Autodesk Inventor part; units mm, degrees
ref_plane "YZ Plane" through (0, 0, 0) normal (1, 0, 0) x (0, 1, 0)
ref_plane "XZ Plane" through (0, 0, 0) normal (0, 1, 0) x (-1, 0, 0)
ref_plane "XY Plane" through (0, 0, 0) normal (0, 0, 1) x (1, 0, 0)
sketch "Sketch1" plane through (0, 0, 0) normal (0, 0, 1) x (1, 0, 0)
  line L0 (-8.9, 0) -> (9.3, 0)
  line L1 (9.3, 0) -> (9.3, -14.13)
  line L2 (-8.9, -14.13) -> (-8.9, 0)
  line L3 (-7.7, -1.2) -> (8.1, -1.2)
  line L4 (8.1, -1.2) -> (8.1, -15.33)
  line L5 (-7.7, -15.33) -> (-7.7, -1.2)
  line L6 (-8.9, -14.13) -> (-17.7, -14.13)
  line L7 (-17.7, -14.13) -> (-17.7, -15.33)
  line L8 (-17.7, -15.33) -> (-7.7, -15.33)
  line L9 (9.3, -14.13) -> (18.1, -14.13)
  line L10 (18.1, -14.13) -> (18.1, -15.33)
  line L11 (18.1, -15.33) -> (8.1, -15.33)
  point P0 (0, 0)
  dimension "d0" = 1.2
  dimension "d1" = 1.2
  dimension "d2" = 1.2
  dimension "d3" = 15.8
  dimension "d4" = 14.13
  dimension "d5" = 10
  dimension "d6" = 10
  dimension "d7" = 1.2
  dimension "d8" = 1.2
extrude "Extrusion1" add sketch "Sketch1" along normal blind 10
sketch "Sketch2" plane through (-17.7, -14.13, 0) normal (0, 1, 0) x (1, 0, 0)
  line L0 (8.8, 0) -> (0, 0)
  line L1 (0, 0) -> (0, -10)
  line L2 (8.8, -10) -> (0, -10)
  line L3 (8.8, 0) -> (8.8, -10)
  point P0 (17.7, 0)
fillet "Fillet1" radius 1 2 edges at (18.1, -14.13, 5) (-17.7, -14.13, 5)
fillet "Fillet2" radius 1.5 4 edges at (-8.9, 0, 5) (9.3, 0, 5) (9.3, -14.13, 5) (-8.9, -14.13, 5)
sketch "Sketch3" plane through (-16.7, -14.13, 10) normal (0, 1, 0) x (1, 0, 0)
  circle A0 centre (3.15, 5) radius 0.5
  line L0 (33.8, 0) -> (27.5, 0)
  line L1 (27.5, 0) -> (27.5, 10)
  line L2 (33.8, 10) -> (27.5, 10)
  line L3 (33.8, 10) -> (33.8, 0)
  line L4 (27.5, 0) -> (27.5, 10)
  line L5 (33.8, 0) -> (27.5, 0)
  line L6 (33.8, 10) -> (33.8, 0)
  line L7 (33.8, 10) -> (27.5, 10)
  line L8 (34.8, 0) -> (33.8, 0)
  line L9 (33.8, 10) -> (34.8, 10)
  line L10 (34.8, 0) -> (34.8, 10)
  line L11 (33.8, 0) -> (34.8, 0)
  line L12 (34.8, 0) -> (34.8, 10)
  line L13 (34.8, 10) -> (33.8, 10)
  line L14 (33.8, 10) -> (33.8, 0)
  line L15 (34.8, 10) -> (34.8, 0)
  line L16 (34.8, 0) -> (34.8, 10)
  line L17 (34.8, 10) -> (34.8, 0)
  circle A1 centre (30.65, 5) radius 0.5
  point P0 (16.7, 10)
  dimension "d16" = 1
  dimension "d17" = 1
extrude "Extrusion2" cut sketch "Sketch3" against normal through all contours A0 | A1
properties part number "Batterijbevestiging"
Input: part model. Units: mm. Frame: model coordinates. A direction names the side the tool comes from. Give positions to 0.01 mm unless a question says otherwise; leave off trailing zeros. Loops run counter-clockwise (first coordinate to the right, second up) from the corner with the lowest first, then second, coordinate; pieces in that order, holes last.
1) Line query: L1, parallel to X at y = -15, z = 5; L2, parallel to X at y = -5.75, z = 8.75; L3, parallel to X at y = -14.75, z = 5. Output: solid intervals per line, ascending.
A:
L1: x = -17.69 to -14.05, -13.05 to -7.7, 8.1 to 13.45, 14.45 to 18.09
L2: x = -8.9 to -7.7, 8.1 to 9.3
L3: x = -17.62 to -14.05, -13.05 to -7.7, 8.1 to 13.45, 14.45 to 18.02
2) Reachability of faces 4 (the flat face through (9.3, -7, 5)), 5 (the flat face through (-7.7, -8, 5)), 6 (the flat face through (-14.2, -14.13, 4.9)), 7 (the flat face through (0, 0, 5)) from +Z, -Z, +X, -X, +Y, -Y: full face, straight path, thin tool, end or side. Return the list, or none.
A:
face 4: +Z, -Z, +X, +Y
face 5: +Z, -Z, -Y
face 6: +Z, -Z, -X, +Y
face 7: +Z, -Z, +X, -X, +Y
3) Section query B-B on y = -8. Return the cut outline in (x, z).
A:
outline: (-8.9, 0) - (-7.7, 0) - (-7.7, 10) - (-8.9, 10) - close; (8.1, 0) - (9.3, 0) - (9.3, 10) - (8.1, 10) - close
4) Section query D-D on x = 10. Return the cut outline in (y, z), and give its area (3 significant figures).
A:
outline: (-15.33, 0) - (-13.9, 0) - (-13.9, 10) - (-15.33, 10) - close
area: 14.3 mm2
5) Section query C-C on z = 8.5. Return the cut outline in (x, y), and give its area (3 significant figures).
A:
outline: (-17.7, -15.33) - (-7.7, -15.33) - (-7.7, -1.2) - (8.1, -1.2) - (8.1, -15.33) - (18.1, -15.33) - (18.1, -15.13) arc R1 ccw to (17.1, -14.13) - (10.8, -14.13) arc R1.5 cw to (9.3, -12.63) - (9.3, -1.5) arc R1.5 ccw to (7.8, 0) - (-7.4, 0) arc R1.5 ccw to (-8.9, -1.5) - (-8.9, -12.63) arc R1.5 cw to (-10.4, -14.13) - (-16.7, -14.13) arc R1 ccw to (-17.7, -15.13) - close
area: 76.4 mm2
6) Section query A-A on x = 13.95. Return the cut outline in (y, z).
A:
outline: (-15.33, 0) - (-14.13, 0) - (-14.13, 4.5) - (-15.33, 4.5) - close; (-15.33, 5.5) - (-14.13, 5.5) - (-14.13, 10) - (-15.33, 10) - close
7) Mould query, pull axis Z, two halves, no side actions, for faces 1 (the flat face through (-8, -8, 0)), 2 (the cylindrical face through (14.427, -14.722, 4.85)), 3 (the flat face through (13, -14.13, 5)). Classes: released by +Z, released by -Z, zero draft, split by the parting line, or undercut.
A:
face 1: released by -Z
face 2: undercut
face 3: zero draft
8) Contact query for flat-ended pins moving along their axis: pin 1 (1.5 mm diameter, centred on y = -10, z = 8, fed in from +X); pin 2 (5 mm diameter, centred on x = -13.5, z = 3, fed in from +Y); pin 3 (5 mm diameter, centred on y = -8, z = 6, fed in from -X). Output: stop coordinate, or through.
A:
pin 1: stops at x = 9.3
pin 2: stops at y = -14.13
pin 3: stops at x = -8.9
